Build history of the part. All positions in model axes, mm. A direction names the side the tool comes from. Round coordinates to 2 decimals unless told otherwise and drop trailing zeros. Write each loop counter-clockwise with the first axis right and the second up, starting at its lowest first coordinate (ties: lowest second). Pieces come first, ordered by that corner, then holes. Notation, with made-up numbers: (73.5, 3.5) -> (125.5, 3.5) arc R18 ccw to (125.5, 30.5) -> close; hole circle Ø8 at (20, 72). An arc over 180 degrees is marked (long way). Return JSON: item names as keys, results as strings.
from build123d import *

# Parameters (mm, degrees)
SKETCH1_R        = 12.7
SKETCH1_R_2      = 1.5
SKETCH1_R_3      = 2.5
EXTRUSION1_DEPTH = 5
SKETCH2_R        = 6
SKETCH2_R_2      = 2.5
EXTRUSION2_DEPTH = 4.2
FILLET1_R        = 0.5


with BuildPart() as part:
    # Sketch1 → Extrusion1 (new body)
    with BuildSketch(Plane(origin=(0, 0, 0), x_dir=(-1, 0, 0), z_dir=(0, 1, 0))):
        with Locations(Location((0, 0, 0), (0, 0, 90))):
            Circle(SKETCH1_R)
        with Locations(Location((-4.75, -8.227241336, 0), (0, 0, 90))):
            Circle(SKETCH1_R_2, mode=Mode.SUBTRACT)
        with Locations(Location((0, 0, 0), (0, 0, 90))):
            Circle(SKETCH1_R_3, mode=Mode.SUBTRACT)
        with Locations(Location((-9.5, 0, 0), (0, 0, 90))):
            Circle(SKETCH1_R_2, mode=Mode.SUBTRACT)
        with Locations(Location((-4.75, 8.227241336, 0), (0, 0, 90))):
            Circle(SKETCH1_R_2, mode=Mode.SUBTRACT)
        with Locations(Location((4.75, 8.227241336, 0), (0, 0, 90))):
            Circle(SKETCH1_R_2, mode=Mode.SUBTRACT)
        with Locations(Location((9.5, 0, 0), (0, 0, 90))):
            Circle(SKETCH1_R_2, mode=Mode.SUBTRACT)
        with Locations(Location((4.75, -8.227241336, 0), (0, 0, 90))):
            Circle(SKETCH1_R_2, mode=Mode.SUBTRACT)
    extrude(amount=EXTRUSION1_DEPTH)

    # Sketch2 → Extrusion2 (add)
    with BuildSketch(Plane(origin=(0, 5, 0), x_dir=(1, 0, 0), z_dir=(0, 1, 0))):
        with Locations(Location((0, 0, 0), (0, 0, 270))):
            Circle(SKETCH2_R)
        with Locations(Location((0, 0, 0), (0, 0, 270))):
            Circle(SKETCH2_R_2, mode=Mode.SUBTRACT)
    extrude(amount=EXTRUSION2_DEPTH)

    # Fillet1
    fillet1_edges = [part.edges().sort_by_distance(p)[0] for p in [
        (0, 0, -12.7),
        (0, 0, -2.5),
        (0, 9.2, -2.5),
        (0, 9.2, -6),
        (0, 5, -12.7),
    ]]
    fillet(fillet1_edges, radius=FILLET1_R)


solid = part.part
Q1. Pin check, flat tips, straight feed: pin 1 Ø3 at (x, z) = (-8.5, 7) entering from -Y; pin 2 Ø1.5 at (x, z) = (9.5, -9) entering from +Y; pin 3 Ø1 at (y, z) = (4, -7) entering from -X; pin 4 Ø5 at (y, z) = (8, -2) entering from -X. Stop position of each tip, or through.
Verdict:
{"pin 1": "stops at y = 0", "pin 2": "stops at y = 4.98", "pin 3": "stops at x = -10.91", "pin 4": "stops at x = -6"}
Q2. Wall check: L1, parallel to X at y = 3.2, z = 0; L2, parallel to Z at x = -4, y = 0.5; L3, parallel to Z at x = -5.75, y = 2.75. Give the ranges that are in metal, low to high.
Verdict:
{"L1": "x = -12.7 to -11, -8 to -2.5, 2.5 to 8, 11 to 12.7", "L2": "z = -12.05 to -9.53, -6.93 to 6.93, 9.53 to 12.05", "L3": "z = -11.32 to -9.35, -7.11 to 7.11, 9.35 to 11.32"}
Q3. Saw through at C-C on z = 8.75. Count the separate pieces of the cut face and the enclosed holes in it, then the cut area to 3 significant figures.
Verdict:
{"separate pieces": "3", "enclosed holes": "0", "area": "63.6 mm²"}
Q4. Two-plate mould, pull along Z, no slides. Class faces 1 (the cylindrical face through (4.175, 2.465, 9.613)), 2 (the cylindrical face through (1.802, 6.824, 5.723)), 3 (the flat face through (-3, 0, 3)): +Z half, -Z half, draft (parallel to the pull), parting line (faces both ways), or undercut.
Verdict:
{"face 1": "undercut", "face 2": "parting line", "face 3": "draft"}
Q5. Saw through at B-B on y = 3. List the corners of the cut face in (x, z).
Verdict:
{"outline": "circle Ø25.4 at (0, 0); hole circle Ø3 at (-9.5, 0); hole circle Ø3 at (-4.75, -8.23); hole circle Ø3 at (-4.75, 8.23); hole circle Ø5 at (0, 0); hole circle Ø3 at (4.75, -8.23); hole circle Ø3 at (4.75, 8.23); hole circle Ø3 at (9.5, 0)"}
Q6. 3-axis set-ups, long thin cutter, end or side, ignore diameter. For faces 4 (the flat face through (6, 5, 3)), 5 (the cylindrical face through (-4.3, 2.46, 9.66)): which of +Z, -Z, +X, -X, +Y, -Y reach the whole face in a straight line?
Verdict:
{"face 4": "+Y", "face 5": "+Y, -Y"}
Q7. Saw through at A-A on x = 0. List the corners of the cut face in (y, z).
Verdict:
{"outline": "(0, -12.2) arc R0.5 ccw to (0.5, -12.7) -> (4.5, -12.7) arc R0.5 ccw to (5, -12.2) -> (5, -6) -> (8.7, -6) arc R0.5 ccw to (9.2, -5.5) -> (9.2, -3) arc R0.5 ccw to (8.7, -2.5) -> (0.5, -2.5) arc R0.5 ccw to (0, -3) -> close; (0, 3) arc R0.5 ccw to (0.5, 2.5) -> (8.7, 2.5) arc R0.5 ccw to (9.2, 3) -> (9.2, 5.5) arc R0.5 ccw to (8.7, 6) -> (5, 6) -> (5, 12.2) arc R0.5 ccw to (4.5, 12.7) -> (0.5, 12.7) arc R0.5 ccw to (0, 12.2) -> close"}
